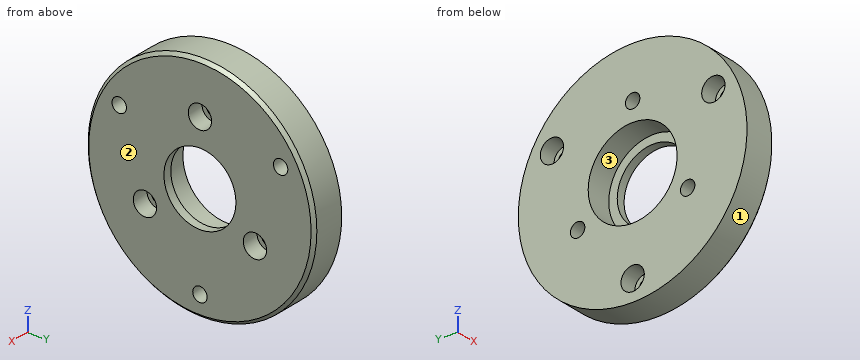
from build123d import *

# Parameters (mm, degrees)
SKETCH046_R         = 27
SKETCH046_R_2       = 8.5
SKETCH046_R_3       = 1.65
PAD029_DEPTH        = 8
SKETCH048_R         = 10.5
POCKET014_DEPTH     = 6
HOLE_D              = 3.4
HOLE_CBORE_D        = 5.5
HOLE_CBORE_DEPTH    = 4
HOLE001_D           = 3.4
HOLE001_CBORE_D     = 5.5
HOLE001_CBORE_DEPTH = 4
CHAMFER_SIZE        = 0.75


with BuildPart() as part:
    # Sketch046 → Pad029 (new body)
    with BuildSketch(Plane.YZ.offset(69)):
        with Locations((-10, -6)):
            Circle(SKETCH046_R)
        with Locations((-10, -6)):
            Circle(SKETCH046_R_2, mode=Mode.SUBTRACT)
        with Locations((-10, 9)):
            Circle(SKETCH046_R_3, mode=Mode.SUBTRACT)
        with Locations((2.990381, -13.5)):
            Circle(SKETCH046_R_3, mode=Mode.SUBTRACT)
        with Locations((-22.990381, -13.5)):
            Circle(SKETCH046_R_3, mode=Mode.SUBTRACT)
    extrude(amount=PAD029_DEPTH)

    # Sketch048 → Pocket014 (cut)
    with BuildSketch(Plane.YZ.offset(69)):
        with Locations((-10, -6)):
            Circle(SKETCH048_R)
    extrude(amount=POCKET014_DEPTH, mode=Mode.SUBTRACT)

    # Hole (through all)
    with Locations(Plane(origin=(69, 0, 0), x_dir=(0, 1, 0), z_dir=(-1, 0, 0))):
        with Locations((-29.052559, -5), (9.052559, -5), (-10, 28)):
            CounterBoreHole(HOLE_D / 2, HOLE_CBORE_D / 2, HOLE_CBORE_DEPTH)

    # Hole001 (through all)
    with Locations(Plane.YZ.offset(77)):
        with Locations((-22.990381, -13.5), (-10, 9), (2.990381, -13.5)):
            CounterBoreHole(HOLE001_D / 2, HOLE001_CBORE_D / 2, HOLE001_CBORE_DEPTH)

    # Chamfer
    chamfer_edges = [part.edges().sort_by_distance(p)[0] for p in [
        (77, -37, -6),
    ]]
    chamfer(chamfer_edges, length=CHAMFER_SIZE)


with BuildPart() as part_1:
    # Body011 placement: moved
    add(part.part.moved(Location((2, -6, 7))))


solid = part_1.part
Work out the finished part from the listing and answer in its coordinate system (mm). Face numbers are marked on the shaded views. Give positions to 0.01 mm unless a question says otherwise; leave off trailing zeros. Order: outer loops, then holes, each group sorted by start corner. A loop starts at its lowest first (then second) coordinate and runs counter-clockwise, first axis right, second up. Notation, with made-up numbers: (-16.5, 60.5) -> (34.5, 60.5) arc R32 ccw to (34.5, 86.5) -> close; hole circle Ø11 at (75.5, 17). An arc over 180 degrees is marked (long way). Answer as a JSON object with one key per item and string values. Group by question number.
1. Section A-A on z = 1 is taken. Determine the outline of the cut face in (x, y).
2. Section C-C on x = 72.25 is taken. Determine the outline of the cut face in (y, z).
3. Consider line 1 along Z through (x, y) = (74, -16); line 2 along Z through (x, y) = (77.6, -16); line 3 along Y through (x, z) = (76.75, 13.5). Determine where each line is inside the solid, lowest interval first. Write a range as [from, to].
4. Section B-B on y = -16 is taken. Count the separate pieces of the cut face and the enclosed holes in it, plus the area to 3 significant figures.
5. Flat-ended cylindrical pins translate along their axes: pin 1 Ø24 at (y, z) = (-16, 1) entering from +X; pin 2 Ø3 at (x, y) = (76, 1) entering from -Z; pin 3 Ø3 at (x, z) = (73, -1.5) entering from -Y; pin 4 Ø4.5 at (y, z) = (-16, 16) entering from +X. Find the tip coordinate at first contact, or state that the pin passes through.
6. The mould has two halves that part along Z. Classify the marked faces 1, 2 and 3: released by +Z, released by -Z, zero draft, split by the parting line, or undercut.
Result sheet:
{
 "1": {"outline": "(71, -43) -> (78.25, -43) -> (79, -42.25) -> (79, -24.5) -> (77, -24.5) -> (77, -26.5) -> (71, -26.5) -> close; (71, -5.5) -> (77, -5.5) -> (77, -7.5) -> (79, -7.5) -> (79, 10.25) -> (78.25, 11) -> (71, 11) -> close"},
 "2": {"outline": "circle Ø54 at (-16, 1); hole circle Ø5.5 at (-35.05, 12); hole circle Ø3.4 at (-28.99, -6.5); hole circle Ø21 at (-16, 1); hole circle Ø5.5 at (-16, -21); hole circle Ø3.4 at (-16, 16); hole circle Ø3.4 at (-3.01, -6.5); hole circle Ø5.5 at (3.05, 12)"},
 "3": {"line 1": "z = [-26, -23.75], [-18.25, -9.5], [11.5, 14.3], [17.7, 28]", "line 2": "z = [-26, -22.7], [-19.3, -7.5], [9.5, 13.25], [18.75, 28]", "line 3": "y = [-39.93, -35.85], [-34.25, -17.15], [-14.85, 2.25], [3.85, 7.93]"},
 "4": {"separate pieces": "4", "enclosed holes": "0", "area": "200 mm^2"},
 "5": {"pin 1": "stops at x = 79", "pin 2": "stops at z = -21.11", "pin 3": "stops at y = -42.98", "pin 4": "stops at x = 75"},
 "6": {"face 1": "split by the parting line", "face 2": "zero draft", "face 3": "undercut"}
}
